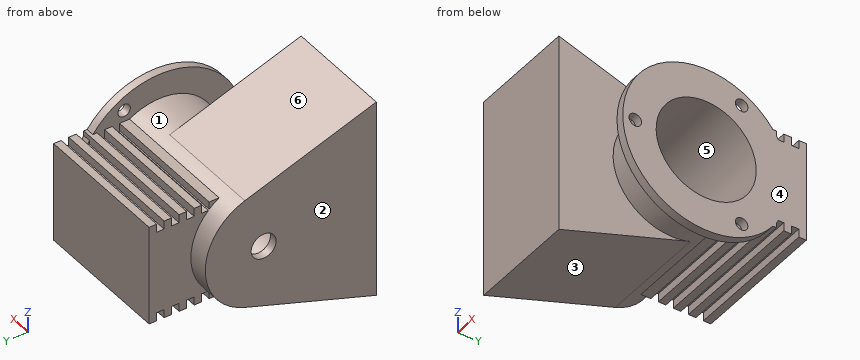
from build123d import *

# Parameters (mm, degrees)
BOSS_EXTRUDE1_DEPTH                                 = 165.1
SKETCH1_3_R                                         = 88.9
BOSS_EXTRUDE2_DEPTH                                 = 228.6
SKETCH2_R                                           = 127
BOSS_EXTRUDE3_DEPTH                                 = 12.7
BOSS_EXTRUDE4_START                                 = -209.55
BOSS_EXTRUDE4_DEPTH                                 = 209.55
CBORE_FOR_00_BINDING_HEAD_MACHINE_SCREW_D           = 38.1
CBORE_FOR_00_BINDING_HEAD_MACHINE_SCREW_CBORE_D     = 152.4
CBORE_FOR_00_BINDING_HEAD_MACHINE_SCREW_CBORE_DEPTH = 228.6
F_97_0_75_DIAMETER_HOLE1_D                          = 19.05
F_97_0_75_DIAMETER_HOLE1_DEPTH                      = 12.7
CIRPATTERN1_COUNT                                   = 3


with BuildPart() as part:
    # Sketch1 → Boss-Extrude1 (new body)
    with BuildSketch(Plane(origin=(0, 0, 0), x_dir=(0, 0, -1), z_dir=(1, 0, 0))):
        with BuildLine():
            Line((-84.14126771, 200.145941668), (-152.4, 0))
            Line((-152.4, 0), (152.4, 0))
            Line((152.4, 0), (84.14126771, 200.145941668))
            ThreePointArc((84.14126771, 200.145941668), (87.702248259, 185.993921421), (88.9, 171.45))
            ThreePointArc((88.9, 171.45), (-14.543921421, 83.747751741), (-84.14126771, 200.145941668))
        make_face()
    extrude(amount=BOSS_EXTRUDE1_DEPTH)

    # Sketch1<3> → Boss-Extrude2 (add)
    with BuildSketch(Plane(origin=(0, 0, 0), x_dir=(0, 0, -1), z_dir=(1, 0, 0))):
        with Locations(Location((0, 171.45, 0), (0, 0, 161.168324383))):
            Circle(SKETCH1_3_R)
    extrude(amount=BOSS_EXTRUDE2_DEPTH)

    # Sketch2 → Boss-Extrude3 (add)
    with BuildSketch(Plane(origin=(228.6, 0, 0), x_dir=(0, 0, -1), z_dir=(1, 0, 0))):
        with Locations((0, 171.45)):
            Circle(SKETCH2_R)
    extrude(amount=BOSS_EXTRUDE3_DEPTH)

    # Sketch3 → Boss-Extrude4 (add)
    with BuildSketch(Plane(origin=(241.3, 0, 0), x_dir=(0, 0, -1), z_dir=(1, 0, 0)).offset(BOSS_EXTRUDE4_START)):
        with BuildLine():
            Line((-76.2, 217.240501198), (-76.2, 232.41))
            Line((-76.2, 232.41), (-64.707715151, 232.41))
            ThreePointArc((-64.707715151, 232.41), (-70.860951664, 225.133661661), (-76.2, 217.240501198))
        make_face()
        with BuildLine():
            Line((-63.5, 233.667039467), (-63.5, 243.84))
            Line((-63.5, 243.84), (-76.2, 243.84))
            Line((-76.2, 243.84), (-76.2, 255.27))
            Line((-76.2, 255.27), (-63.5, 255.27))
            Line((-63.5, 255.27), (-63.5, 266.7))
            Line((-63.5, 266.7), (-76.2, 266.7))
            Line((-76.2, 266.7), (-76.2, 278.13))
            Line((-76.2, 278.13), (-63.5, 278.13))
            Line((-63.5, 278.13), (-63.5, 289.56))
            Line((-63.5, 289.56), (-76.2, 289.56))
            Line((-76.2, 289.56), (-76.2, 300.99))
            Line((-76.2, 300.99), (-63.5, 300.99))
            Line((-63.5, 300.99), (-63.5, 312.42))
            Line((-63.5, 312.42), (-76.2, 312.42))
            Line((-76.2, 312.42), (-76.2, 323.85))
            Line((-76.2, 323.85), (76.2, 323.85))
            Line((76.2, 323.85), (76.2, 312.42))
            Line((76.2, 312.42), (63.5, 312.42))
            Line((63.5, 312.42), (63.5, 300.99))
            Line((63.5, 300.99), (76.2, 300.99))
            Line((76.2, 300.99), (76.2, 289.56))
            Line((76.2, 289.56), (63.5, 289.56))
            Line((63.5, 289.56), (63.5, 278.13))
            Line((63.5, 278.13), (76.2, 278.13))
            Line((76.2, 278.13), (76.2, 266.7))
            Line((76.2, 266.7), (63.5, 266.7))
            Line((63.5, 266.7), (63.5, 255.27))
            Line((63.5, 255.27), (76.2, 255.27))
            Line((76.2, 255.27), (76.2, 243.84))
            Line((76.2, 243.84), (63.5, 243.84))
            Line((63.5, 243.84), (63.5, 233.667039467))
            ThreePointArc((63.5, 233.667039467), (0, 260.35), (-63.5, 233.667039467))
        make_face()
        with BuildLine():
            Line((76.2, 217.240501198), (76.2, 232.41))
            Line((76.2, 232.41), (64.707715151, 232.41))
            ThreePointArc((64.707715151, 232.41), (70.860951664, 225.133661661), (76.2, 217.240501198))
        make_face()
    extrude(amount=BOSS_EXTRUDE4_DEPTH)

    # CBORE for #00 Binding Head Machine Screw1 (through all)
    with Locations(Plane(origin=(241.3, 0, 0), x_dir=(0, 0, -1), z_dir=(1, 0, 0))):
        with Locations((0, 171.45)):
            CounterBoreHole(CBORE_FOR_00_BINDING_HEAD_MACHINE_SCREW_D / 2, CBORE_FOR_00_BINDING_HEAD_MACHINE_SCREW_CBORE_D / 2, CBORE_FOR_00_BINDING_HEAD_MACHINE_SCREW_CBORE_DEPTH)

    # #97 (0.75) Diameter Hole1
    with Locations(Plane(origin=(241.3, 0, 0), x_dir=(0, 0, -1), z_dir=(1, 0, 0))):
        with Locations((0, 63.5)):
            f_97_0_75_diameter_hole1 = Hole(F_97_0_75_DIAMETER_HOLE1_D / 2, depth=F_97_0_75_DIAMETER_HOLE1_DEPTH)

    # CirPattern1: #97 (0.75) Diameter Hole1 ×3 about axis
    cirpattern1_axis = Axis((0, 171.45, 0), (1, 0, 0))
    for i in range(1, CIRPATTERN1_COUNT):
        add(f_97_0_75_diameter_hole1.rotate(cirpattern1_axis, i * 360 / CIRPATTERN1_COUNT), mode=Mode.SUBTRACT)


solid = part.part
The listing builds one solid part. Answer for the finished solid, in the listing's coordinates (mm). Face numbers are marked on the shaded views. A direction names the side the tool comes from. Coordinates: 2 decimals unless noted, no trailing zeros. Order: outer loops, then holes, each group sorted by start corner. A loop starts at its lowest first (then second) coordinate and runs counter-clockwise, first axis right, second up. Notation, with made-up numbers: M -33,72.25 L 26,72.25 A30 cw 26,106.25 Z; hole C 48.25,-36.5 d1. An arc over 180 degrees is marked long. Use CSV: the item, a comma, the result in double quotes.
Q1. Section C-C (y = 171.45) is taken. Determine the outline of the cut face in (x, z).
Here are the results:
outline,"M 0,-93.93 L 165.1,-93.93 L 165.1,-88.9 L 228.6,-88.9 L 228.6,-127 L 241.3,-127 L 241.3,-76.2 L 12.7,-76.2 L 12.7,-19.05 L 0,-19.05 Z; M 0,19.05 L 12.7,19.05 L 12.7,76.2 L 241.3,76.2 L 241.3,127 L 228.6,127 L 228.6,88.9 L 165.1,88.9 L 165.1,93.93 L 0,93.93 Z"
Q2. Section B-B (z = -109) is taken. Determine the outline of the cut face in (x, y), then the cut area to 3 significant figures.
Here are the results:
outline,"M 0,0 L 165.1,0 L 165.1,127.26 L 0,127.26 Z; M 228.6,106.27 L 241.3,106.27 L 241.3,236.63 L 228.6,236.63 Z"
area,"22,700 mm2"
Q3. Determine the mould class of the marked faces 1, 2 and 3 for opening direction X: pulls with the +X half, pulls with the -X half, needs draft (parallel to the pull), parting line crosses it, or undercut.
Here are the results:
face 1,"undercut"
face 2,"pulls with the -X half"
face 3,"needs draft"
Q4. Given pin 1 Ø9 at (x, y) = (175.5, 320.5) entering from +Z; pin 2 Ø1 at (y, z) = (39, -119) entering from +X; pin 3 Ø5.5 at (x, y) = (117.5, 305.5) entering from -Z, each flat-ended and moving along its own axis, determine where each tip first touches the part or whether it passes through.
Here are the results:
pin 1,"z = 76.2"
pin 2,"x = 165.1"
pin 3,"z = -63.5"
Q5. Section A-A (y = 227.5) is taken. Determine the outline of the cut face in (x, z), then the cut area to 3 significant figures.
Here are the results:
outline,"M 0,-69 L 31.75,-69 L 31.75,-76.2 L 228.6,-76.2 L 228.6,-84.19 L 241.3,-84.19 L 241.3,-51.62 L 12.7,-51.62 L 12.7,51.62 L 241.3,51.62 L 241.3,84.19 L 228.6,84.19 L 228.6,76.2 L 31.75,76.2 L 31.75,69 L 0,69 Z; M 228.6,-113.96 L 241.3,-113.96 L 241.3,-102.78 L 228.6,-102.78 Z; M 228.6,102.78 L 241.3,102.78 L 241.3,113.96 L 228.6,113.96 Z"
area,"13,200 mm2"
Q6. Section D-D (z = -5) is taken. Determine the outline of the cut face in (x, y), then the cut area to 3 significant figures.
Here are the results:
outline,"M 0,0 L 165.1,0 L 165.1,82.69 L 228.6,82.69 L 228.6,71.61 L 241.3,71.61 L 241.3,95.41 L 12.7,95.41 L 12.7,153.07 L 0,153.07 Z; M 0,189.83 L 12.7,189.83 L 12.7,247.49 L 241.3,247.49 L 241.3,323.85 L 31.75,323.85 L 31.75,260.21 L 0,260.21 Z; M 228.6,44.55 L 241.3,44.55 L 241.3,55.39 L 228.6,55.39 Z"
area,"34,900 mm2"
Q7. A tool of negligible diameter and unlimited length cuts with its end or side. For the marked faces 4, 5 and 6, from which of +Z, -Z, +X, -X, +Y, -Y can it reach the whole face along a straight path? Write none if from no direction.
Here are the results:
face 4,"+Z, -Z, +X, +Y, -Y"
face 5,"+X"
face 6,"+Z, -X, +Y"
Q8. Straight lines are drawn through the part: L1, parallel to Y at x = 238, z = 0 (3 decimals); L2, parallel to Y at x = 133, z = 0; L3, parallel to Y at x = 196, z = 2.5. For each, find the intervals that lie inside material, in ascending order.
Here are the results:
L1,"44.45 to 53.975, 73.025 to 95.25, 247.65 to 323.85"
L2,"0 to 95.25, 247.65 to 323.85"
L3,"82.59 to 95.29, 247.61 to 323.85"
